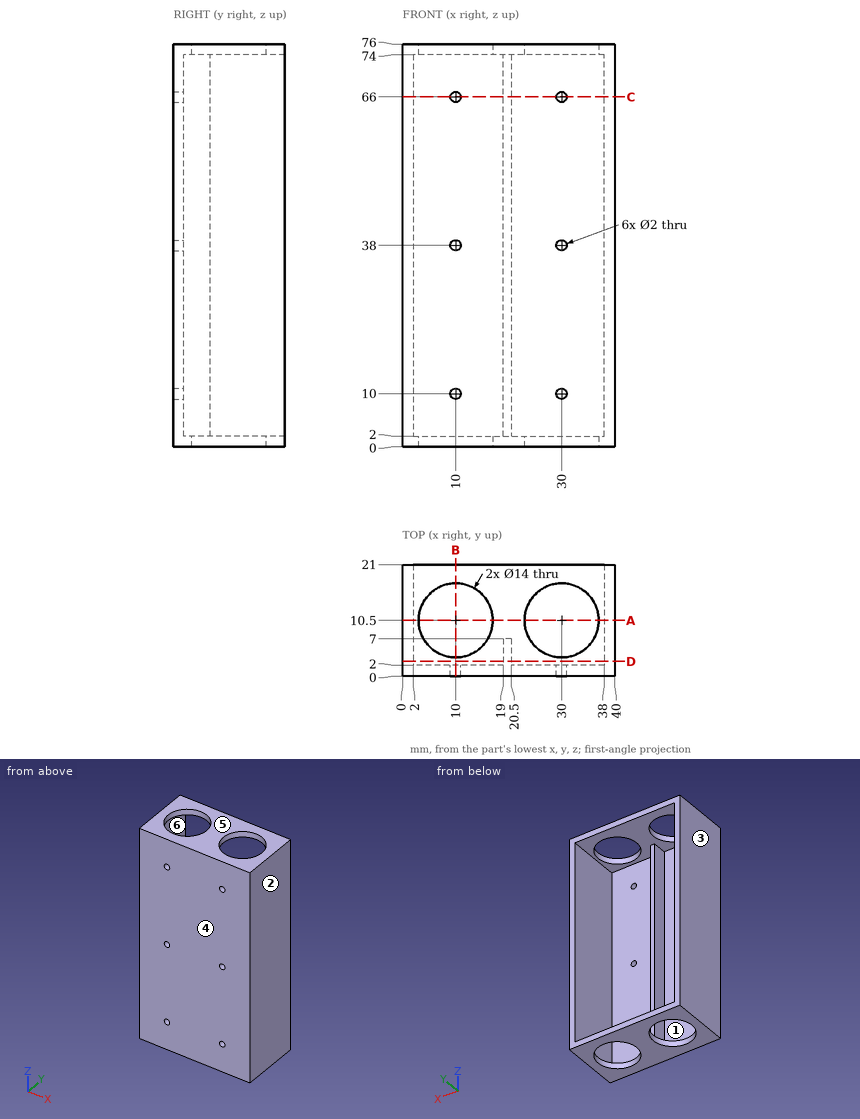
Answer from the drawing. Dimensions are ordinates in mm from the lowest x, y and z of the part. A direction names the side the tool comes from. Give positions to 0.01 mm unless a question says otherwise; leave off trailing zeros. Write each loop counter-clockwise with the first axis right and the second up, starting at its lowest first coordinate (ties: lowest second). Pieces come first, ordered by that corner, then holes. Notation, with made-up numbers: (-0.75, 28) -> (28.25, 28) arc R28 cw to (28.25, 67) -> close; hole circle Ø2 at (26, -18.5). An arc over 180 degrees is marked (long way). One line per question, with ' | ' between items. Start each with the question number.
1. Given pin 1 Ø2.5 at (x, z) = (10, 66) entering from +Y; pin 2 Ø1.2 at (x, z) = (10, 10) entering from -Y; pin 3 Ø18.5 at (x, z) = (13.5, 21.5) entering from +Y; pin 4 Ø1.5 at (x, z) = (9.5, 47) entering from -Y, each flat-ended and moving along its own axis, determine where each tip first touches the part or whether it passes through.
2. Section B-B (x = 10) is taken. Determine the outline of the cut face in (y, z).
3. Section A-A (y = 10.5) is taken. Determine the outline of the cut face in (x, z), plus the area to 3 significant figures.
4. For a pull along X with two mould halves and no side action, classify the marked faces 1, 2, 3 and 4 as pulls with the +X half, pulls with the -X half, needs draft (parallel to the pull), parting line crosses it, or undercut.
5. Section D-D (y = 2.75) is taken. Determine the outline of the cut face in (x, z), plus the area to 3 significant figures.
6. For the marked faces 5 and 6, determine the directions among +Z, -Z, +X, -X, +Y, -Y from which every point of the face is accessible in a straight line to the end or side of a thin tool.
7. Find the intervals of material crossed by probe 1 along Z at (x, y) = (30, 0.7); probe 2 along X at (y, z) = (4, 15); probe 3 along X at (y, z) = (10.5, 1.35), in increasing order.
8. Section C-C (z = 66) is taken. Determine the outline of the cut face in (x, y), plus the area to 4 significant figures.
Response values:
1) pin 1: y = 2 | pin 2: through | pin 3: y = 7 | pin 4: y = 0
2) outline: (0, 0) -> (3.5, 0) -> (3.5, 2) -> (2, 2) -> (2, 9) -> (0, 9) -> close; (0, 11) -> (2, 11) -> (2, 37) -> (0, 37) -> close; (0, 39) -> (2, 39) -> (2, 65) -> (0, 65) -> close; (0, 67) -> (2, 67) -> (2, 74) -> (3.5, 74) -> (3.5, 76) -> (0, 76) -> close; (17.5, 0) -> (21, 0) -> (21, 2) -> (17.5, 2) -> close; (17.5, 74) -> (21, 74) -> (21, 76) -> (17.5, 76) -> close
3) outline: (0, 0) -> (3, 0) -> (3, 2) -> (2, 2) -> (2, 74) -> (3, 74) -> (3, 76) -> (0, 76) -> close; (17, 0) -> (23, 0) -> (23, 2) -> (17, 2) -> close; (17, 74) -> (23, 74) -> (23, 76) -> (17, 76) -> close; (37, 0) -> (40, 0) -> (40, 76) -> (37, 76) -> (37, 74) -> (38, 74) -> (38, 2) -> (37, 2) -> close | area: 336 mm2
4) face 1: undercut | face 2: pulls with the +X half | face 3: pulls with the -X half | face 4: needs draft
5) outline: (0, 0) -> (40, 0) -> (40, 76) -> (0, 76) -> close; hole (2, 2) -> (19, 2) -> (19, 74) -> (2, 74) -> close; hole (20.5, 2) -> (38, 2) -> (38, 74) -> (20.5, 74) -> close | area: 556 mm2
6) face 5: +Z, +X, -X, +Y, -Y | face 6: +Y
7) probe 1: 0 to 9, 11 to 37, 39 to 65, 67 to 76 | probe 2: 0 to 2, 19 to 20.5, 38 to 40 | probe 3: 0 to 3, 17 to 23, 37 to 40
8) outline: (0, 0) -> (9, 0) -> (9, 2) -> (2, 2) -> (2, 21) -> (0, 21) -> close; (11, 0) -> (29, 0) -> (29, 2) -> (20.5, 2) -> (20.5, 7) -> (19, 7) -> (19, 2) -> (11, 2) -> close; (31, 0) -> (40, 0) -> (40, 21) -> (38, 21) -> (38, 2) -> (31, 2) -> close | area: 155.5 mm2
